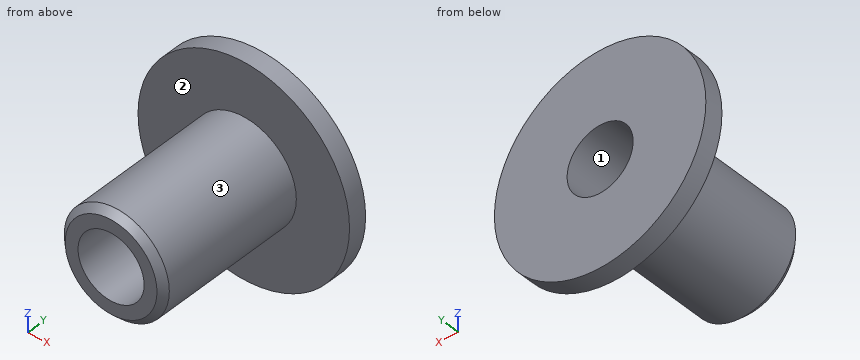
from build123d import *

# Parameters (mm, degrees)
F0_R     = 7.95
F0_R_2   = 5
F1_DEPTH = 26
F0_R_3   = 16
F2_DEPTH = 2.81
F3_SIZE  = 1


with BuildPart() as f1:
    # F0 (on Front) → F1 (new body)
    with BuildSketch(Plane.XZ):
        Circle(F0_R)
        Circle(F0_R_2, mode=Mode.SUBTRACT)
    extrude(amount=F1_DEPTH)

    # F0 (on Front) → F2 (join)
    with BuildSketch(Plane.XZ):
        Circle(F0_R_3)
        Circle(F0_R, mode=Mode.SUBTRACT)
    extrude(amount=F2_DEPTH)

    # F3
    f3_edges = [f1.edges().sort_by_distance(p)[0] for p in [
        (-7.95, -26, 0),
    ]]
    chamfer(f3_edges, length=F3_SIZE)


solid = f1.part
Can you work these out from the model? Positions are in its coordinate system, mm. Face numbers are marked on the shaded views. Coordinates: 2 decimals unless noted, no trailing zeros. Loops run counter-clockwise (first coordinate to the right, second up) from the corner with the lowest first, then second, coordinate; pieces in that order, holes last. Notation, with made-up numbers: M 62,81 L 110,81 A21 ccw 110,112 Z; hole C 42.25,-7 d10. An arc over 180 degrees is marked long. Return JSON: item names as keys, results as strings. Group by question number.
Item 1: Imagine slicing it at C-C (y = -2.25). Please give me the cut outline in (x, z), and give its area (3 significant figures).
Item 2: Thinking about a two-plate mould opening in X: for the marked faces 1, 2 and 3, which applies, released by +X, released by -X, zero draft, split by the parting line, or undercut?
Item 3: If I drill on L1, parallel to Z at x = 0, y = -18.75; L2, parallel to Y at x = -8, z = 12; L3, parallel to Z at x = 1.5, y = -15.75, over which ranges is the centre line in solid material (lowest first)? Write a range as from..to.
Item 4: I'm going to push flat-ended pins straight in: pin 1 Ø10 at (x, y) = (-5.5, -17) entering from -Z; pin 2 Ø12 at (x, y) = (-2, -12.5) entering from +Z; pin 3 Ø2 at (y, z) = (-16.5, 5) entering from +X; pin 4 Ø1 at (y, z) = (-17.5, -10) entering from -X. Where does each tip first touch, or does it pass through?
Item 5: Imagine slicing it at D-D (z = 10). Please give me the cut outline in (x, y), and give its area (3 significant figures).
Item 6: Imagine slicing it at A-A (x = 0). Please give me the cut outline in (y, z), and give its area (3 significant figures).
Item 7: Imagine slicing it at B-B (z = 0). Please give me the cut outline in (x, y), and give its area (3 significant figures).
Verdict:
{
 "1": {"outline": "C 0,0 d32; hole C 0,0 d10", "area": "726 mm^2"},
 "2": {"face 1": "undercut", "face 2": "zero draft", "face 3": "split by the parting line"},
 "3": {"L1": "z = -7.95..-5, 5..7.95", "L2": "y = -2.81..0", "L3": "z = -7.81..-4.77, 4.77..7.81"},
 "4": {"pin 1": "stops at z = -7.93", "pin 2": "stops at z = 7.95", "pin 3": "stops at x = 6.87", "pin 4": "passes through"},
 "5": {"outline": "M -12.49,-2.81 L 12.49,-2.81 L 12.49,0 L -12.49,0 Z", "area": "70.2 mm^2"},
 "6": {"outline": "M -26,-6.95 L -25,-7.95 L -2.81,-7.95 L -2.81,-16 L 0,-16 L 0,-5 L -26,-5 Z; M -26,5 L 0,5 L 0,16 L -2.81,16 L -2.81,7.95 L -25,7.95 L -26,6.95 Z", "area": "198 mm^2"},
 "7": {"outline": "M -16,-2.81 L -7.95,-2.81 L -7.95,-25 L -6.95,-26 L -5,-26 L -5,0 L -16,0 Z; M 5,-26 L 6.95,-26 L 7.95,-25 L 7.95,-2.81 L 16,-2.81 L 16,0 L 5,0 Z", "area": "198 mm^2"}
}
